For this review, take the finished solid that the model builds, in its own axes (mm). Face numbers are marked on the shaded views. A direction names the side the tool comes from. Coordinates: 2 decimals unless noted, no trailing zeros. Loops run counter-clockwise (first coordinate to the right, second up) from the corner with the lowest first, then second, coordinate; pieces in that order, holes last. Notation, with made-up numbers: M -30,43 L 18,43 A14 ccw 18,55 Z; hole C 58.5,-33.5 d11. An arc over 180 degrees is marked long. Answer as a JSON object with one key per item and string values. Group by question number.
Item 1: Insertion check: pin 1 (4 mm diameter, centred on y = 1.5, z = 0, fed in from -X); pin 2 (8 mm diameter, centred on x = 48.5, z = -1.5, fed in from -Y); pin 3 (4 mm diameter, centred on y = 9, z = 15, fed in from -X); pin 4 (4 mm diameter, centred on y = 3.5, z = 2.5, fed in from +X). Each pin has a flat end and moves straight along its axis. Give the tip position at first contact, or say it passes through.
Item 2: Wall thickness on L1, parallel to Y at x = 69.25, z = 15; L2, parallel to X at y = 2.5, z = 3.5; L3, parallel to Z at x = 44, y = 6: over which ranges is each line inside the solid? List them lowest first. Write a range as from..to.
Item 3: Add section D-D (x = 37). State the section outline as (y, z) points, then the cut area to 3 significant figures.
Item 4: Add section A-A (y = 2.25). State the section outline as (x, z) points.
Item 5: Add section B-B (y = 9). State the section outline as (x, z) points.
Item 6: Add section C-C (z = 2.5). State the section outline as (x, y) points.
Item 7: Mouldability with a two-part tool opening along X and no side actions: class the marked faces 1, 2 and 3 as +X half, -X half, draft (parallel to the pull), parting line (faces both ways), or undercut.
Item 8: Tool access review of the marked faces 4, 5, 6, 7 and 8: name each direction out of +Z, -Z, +X, -X, +Y, -Y from which nothing blocks a thin tool from reaching the whole face with its end or side.
from build123d import *

# Parameters (mm, degrees)
MAIN_DEPTH             = 5
MAKERBEAMFIX_DEPTH     = 20
SKETCH2_R              = 1.5
MAKERBEAMFIXHOLE_DEPTH = 30
FILLET1_R              = 5


with BuildPart() as part:
    # Esquisse1 → Main (new body, symmetric)
    with BuildSketch(Plane.XY):
        Polygon((3, 0), (3, 5), (15, 5), (15, 0), (22, 0), (22, 5), (34, 5), (34, 0), (41, 0), (41, 5), (53, 5), (53, 0), (60, 0), (60, 5), (71, 5), (71, 8), (0, 8), (0, 0), align=None)
    extrude(amount=MAIN_DEPTH, both=True)

    # Sketch1 → MakerBeamFix (add, symmetric)
    with BuildSketch(Plane.XY):
        Polygon((66, 14), (71, 14), (71, 10.45), (72, 10.45), (72, 7.55), (71, 7.55), (71, 5), (66, 5), align=None)
    extrude(amount=MAKERBEAMFIX_DEPTH, both=True)

    # Sketch2 → MakerBeamFixHole (cut)
    with BuildSketch(Plane(origin=(72, 0, 0), x_dir=(0, 0, -1), z_dir=(1, 0, 0))):
        with Locations((-15, 9)):
            Circle(SKETCH2_R)
        with Locations((15, 9)):
            Circle(SKETCH2_R)
    extrude(amount=-MAKERBEAMFIXHOLE_DEPTH, mode=Mode.SUBTRACT)

    # Fillet1
    fillet1_edges = [part.edges().sort_by_distance(p)[0] for p in [
        (66, 6.5, -5),
        (66, 6.5, 5),
        (66, 8, 0),
    ]]
    fillet(fillet1_edges, radius=FILLET1_R)


solid = part.part
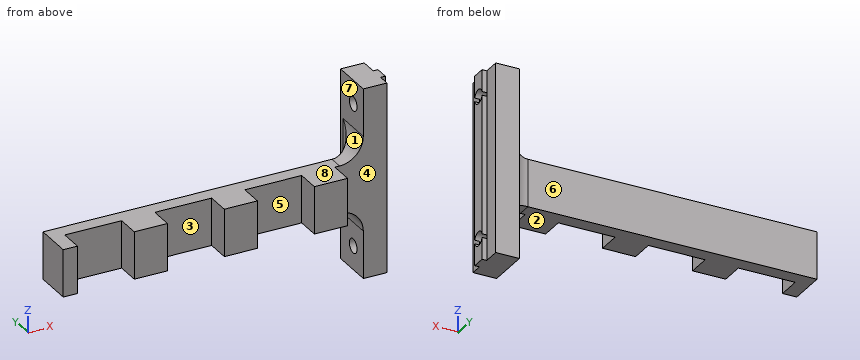
From the geometry:
{
 "1": {"pin 1": "stops at x = 0", "pin 2": "stops at y = 5", "pin 3": "stops at x = 66", "pin 4": "stops at x = 71"},
 "2": {"L1": "y = 5..7.5, 10.5..14", "L2": "x = 0..3, 15..22, 34..41, 53..60", "L3": "z = -5..5"},
 "3": {"outline": "M 0,-5 L 8,-5 L 8,5 L 0,5 Z", "area": "80.0 mm²"},
 "4": {"outline": "M 0,-5 L 3,-5 L 3,5 L 0,5 Z; M 15,-5 L 22,-5 L 22,5 L 15,5 Z; M 34,-5 L 41,-5 L 41,5 L 34,5 Z; M 53,-5 L 60,-5 L 60,5 L 53,5 Z"},
 "5": {"outline": "M 64,-6 A5 cw 66,-10 L 66,-13.5 L 72,-13.5 L 72,13.5 L 66,13.5 L 66,10 A5 cw 64,6 Z; M 66,-20 L 72,-20 L 72,-16.5 L 66,-16.5 Z; M 66,16.5 L 72,16.5 L 72,20 L 66,20 Z"},
 "6": {"outline": "M 0,0 L 3,0 L 3,5 L 15,5 L 15,0 L 22,0 L 22,5 L 34,5 L 34,0 L 41,0 L 41,5 L 53,5 L 53,0 L 60,0 L 60,5 L 71,5 L 71,7.55 L 72,7.55 L 72,10.45 L 71,10.45 L 71,14 L 66,14 L 66,13 A5 cw 61,8 L 0,8 Z"},
 "7": {"face 1": "-X half", "face 2": "draft", "face 3": "undercut"},
 "8": {"face 4": "+Z, -Z, +X, -Y", "face 5": "+Z, -Z, -Y", "face 6": "+Z, -Z, -X, +Y", "face 7": "-X, +Y", "face 8": "+Z, -X, +Y, -Y"}
}
